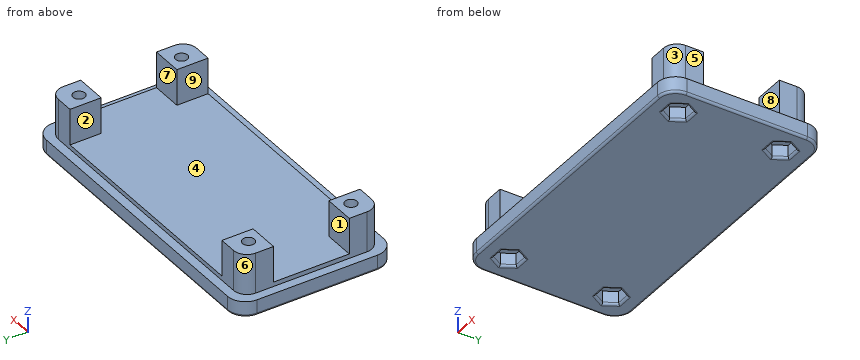
```python
from build123d import *

# Parameters (mm, degrees)
F1_DEPTH = 3.5
F3_DEPTH = 1
F5_DEPTH = 8.1
F6_R     = 1.35
F7_DEPTH = 3
F8_DEPTH = 12.601
F9_R     = 0.5


with BuildPart() as f1:
    # F0 (on Top) → F1 (new body)
    with BuildSketch(Plane.XY):
        with BuildLine():
            Line((31, 17.5), (-31, 17.5))
            ThreePointArc((-31, 17.5), (-33.8284271247, 16.3284271247), (-35, 13.5))
            Line((-35, 13.5), (-35, -13.5))
            ThreePointArc((-35, -13.5), (-33.8284271247, -16.3284271247), (-31, -17.5))
            Line((-31, -17.5), (31, -17.5))
            ThreePointArc((31, -17.5), (33.8284271247, -16.3284271247), (35, -13.5))
            Line((35, -13.5), (35, 13.5))
            ThreePointArc((35, 13.5), (33.8284271247, 16.3284271247), (31, 17.5))
        make_face()
    extrude(amount=F1_DEPTH)

    # F2 (on face) → F3 (join)
    with BuildSketch(Plane.XY.offset(3.5)):
        with BuildLine():
            Line((29.9999990687, 15.5), (-30.0000009313, 15.5))
            ThreePointArc((-30.0000009313, 15.5), (-32.1213212749, 14.6213203436), (-33.0000009313, 12.5))
            Line((-33.0000009313, 12.5), (-33.0000009313, -12.5))
            ThreePointArc((-33.0000009313, -12.5), (-32.1213212749, -14.6213203436), (-30.0000009313, -15.5))
            Line((-30.0000009313, -15.5), (29.9999990687, -15.5))
            ThreePointArc((29.9999990687, -15.5), (32.1213194122, -14.6213203436), (32.9999990687, -12.5))
            Line((32.9999990687, -12.5), (32.9999990687, 12.5))
            ThreePointArc((32.9999990687, 12.5), (32.1213194122, 14.6213203436), (29.9999990687, 15.5))
        make_face()
    extrude(amount=F3_DEPTH)

    # F4 (on face) → F5 (join)
    with BuildSketch(Plane.XY.offset(4.5)):
        with BuildLine():
            Line((-26, 15.5), (-30.0000009313, 15.5))
            ThreePointArc((-30.0000009313, 15.5), (-32.1213212749, 14.6213203436), (-33.0000009313, 12.5))
            Line((-33.0000009313, 12.5), (-33.0000009313, 8.5))
            Line((-33.0000009313, 8.5), (-26, 8.5))
            Line((-26, 8.5), (-26, 15.5))
        make_face()
        with BuildLine():
            Line((-26, -8.5), (-33.0000009313, -8.5))
            Line((-33.0000009313, -8.5), (-33.0000009313, -12.5))
            ThreePointArc((-33.0000009313, -12.5), (-32.1213212749, -14.6213203436), (-30.0000009313, -15.5))
            Line((-30.0000009313, -15.5), (-26, -15.5))
            Line((-26, -15.5), (-26, -8.5))
        make_face()
        with BuildLine():
            Line((29.9999990687, 15.5), (26, 15.5))
            Line((26, 15.5), (26, 8.5))
            Line((26, 8.5), (32.9999990687, 8.5))
            Line((32.9999990687, 8.5), (32.9999990687, 12.5))
            ThreePointArc((32.9999990687, 12.5), (32.1213194122, 14.6213203436), (29.9999990687, 15.5))
        make_face()
        with BuildLine():
            Line((32.9999990687, -12.5), (32.9999990687, -8.5))
            Line((32.9999990687, -8.5), (26, -8.5))
            Line((26, -8.5), (26, -15.5))
            Line((26, -15.5), (29.9999990687, -15.5))
            ThreePointArc((29.9999990687, -15.5), (32.1213194122, -14.6213203436), (32.9999990687, -12.5))
        make_face()
    extrude(amount=F5_DEPTH)

    # F6 (on face) → F7 (cut)
    with BuildSketch(Plane(origin=(0, 0, 0), x_dir=(1, 0, 0), z_dir=(0, 0, -1))):
        Polygon((-30.5011106999, 8.9), (-27.4988893001, 8.9), (-25.9977786002, 11.5), (-27.4988893001, 14.1), (-30.5011106999, 14.1), (-32.0022213998, 11.5), align=None)
        with Locations((-29, 11.5)):
            Circle(F6_R, mode=Mode.SUBTRACT)
        Polygon((27.4988893001, 8.9), (30.5011106999, 8.9), (32.0022213998, 11.5), (30.5011106999, 14.1), (27.4988893001, 14.1), (25.9977786002, 11.5), align=None)
        with Locations((29, 11.5)):
            Circle(F6_R, mode=Mode.SUBTRACT)
        Polygon((30.5011106999, -8.9), (27.4988893001, -8.9), (25.9977786002, -11.5), (27.4988893001, -14.1), (30.5011106999, -14.1), (32.0022213998, -11.5), align=None)
        with Locations((29, -11.5)):
            Circle(F6_R, mode=Mode.SUBTRACT)
        Polygon((-27.4988893001, -8.9), (-30.5011106999, -8.9), (-32.0022213998, -11.5), (-30.5011106999, -14.1), (-27.4988893001, -14.1), (-25.9977786002, -11.5), align=None)
        with Locations((-29, -11.5)):
            Circle(F6_R, mode=Mode.SUBTRACT)
    extrude(amount=-F7_DEPTH, mode=Mode.SUBTRACT)

    # F8 (cut, through all): faces of the model
    f8_faces = [f1.faces().sort_by_distance(p)[0] for p in [
        (-29, -11.5, 0),
        (29, -11.5, 0),
        (29, 11.5, 0),
        (-29, 11.5, 0),
    ]]
    extrude(f8_faces, amount=-F8_DEPTH, mode=Mode.SUBTRACT)

    # F9
    f9_edges = [f1.edges().sort_by_distance(p)[0] for p in [
        (0, 17.5, 0),
        (33.828427, 16.328427, 0),
        (-33.828427, 16.328427, 0),
        (35, 0, 0),
        (-35, 0, 0),
        (33.828427, -16.328427, 0),
        (-33.828427, -16.328427, 0),
        (0, -17.5, 0),
        (-31.251666, -12.8, 0),
        (-29, -14.1, 0),
        (-26.748334, -12.8, 0),
        (-26.748334, -10.2, 0),
        (-29, -8.9, 0),
        (-31.251666, -10.2, 0),
        (26.748334, -10.2, 0),
        (26.748334, -12.8, 0),
        (29, -14.1, 0),
        (31.251666, -12.8, 0),
        (31.251666, -10.2, 0),
        (29, -8.9, 0),
        (-26.748334, 10.2, 0),
        (-26.748334, 12.8, 0),
        (-29, 14.1, 0),
        (-31.251666, 12.8, 0),
        (-31.251666, 10.2, 0),
        (-29, 8.9, 0),
        (31.251666, 10.2, 0),
        (31.251666, 12.8, 0),
        (29, 14.1, 0),
        (26.748334, 12.8, 0),
        (26.748334, 10.2, 0),
        (29, 8.9, 0),
    ]]
    fillet(f9_edges, radius=F9_R)


solid = f1.part
```
Check sheet for the modelled part. Datum: model origin and axes. Units: mm. Face numbers are marked on the shaded views. A direction names the side the tool comes from. Round coordinates to 2 decimals unless told otherwise and drop trailing zeros. Order: outer loops, then holes, each group sorted by start corner. A loop starts at its lowest first (then second) coordinate and runs counter-clockwise, first axis right, second up.
1) Section check C-C (y = 7.5). Record the boundary of the cut face in (x, z).
2) Section check A-A (z = 5.5). Record the boundary of the cut face in (x, y).
3) Mould release check, pull along Y, two halves, no side actions. Record for the marked faces 6, 7, 8 and 9: +Y half, -Y half, draft (parallel to the pull), parting line (faces both ways), or undercut.
4) Scan lines: line 1 (Y direction, x = -29.5, z = 0.5); line 2 (Y direction, x = -29, z = 5.5); line 3 (X direction, y = -11.5, z = 5.75). Record each from-to range of solid material in increasing order.
5) Tool access check on the marked faces 1, 2, 3, 4 and 5. Record the directions out of +Z, -Z, +X, -X, +Y, -Y that give a thin tool (end or side, any length) a straight path to the whole face; none if there is none.
6) Section check B-B (x = -29). Give the number of separate pieces and of enclosed holes in the cut face, and give its area (3 significant figures).
7) Go/stop test with flat-tipped pins: pin 1 Ø2 at (x, z) = (28, 8) entering from -Y; pin 2 Ø2 at (y, z) = (12, 9) entering from +X; pin 3 Ø2.5 at (x, y) = (-27.5, -11.5) entering from -Z. Record where each tip stops, or that it passes through.
Result:
1. outline: (-35, 0.5) arc R0.5 ccw to (-34.5, 0) - (34.5, 0) arc R0.5 ccw to (35, 0.5) - (35, 3.5) - (33, 3.5) - (33, 4.5) - (-33, 4.5) - (-33, 3.5) - (-35, 3.5) - close
2. outline: (-33, -12.5) arc R3 ccw to (-30, -15.5) - (-26, -15.5) - (-26, -8.5) - (-33, -8.5) - close; (-33, 8.5) - (-26, 8.5) - (-26, 15.5) - (-30, 15.5) arc R3 ccw to (-33, 12.5) - close; (26, -15.5) - (30, -15.5) arc R3 ccw to (33, -12.5) - (33, -8.5) - (26, -8.5) - close; (26, 8.5) - (33, 8.5) - (33, 12.5) arc R3 ccw to (30, 15.5) - (26, 15.5) - close; hole circle Ø2.7 at (-29, -11.5); hole circle Ø2.7 at (-29, 11.5); hole circle Ø2.7 at (29, -11.5); hole circle Ø2.7 at (29, 11.5)
3. face 6: +Y half
3. face 7: undercut
3. face 8: undercut
3. face 9: draft
4. line 1: y = -17.5 to -14.1, -8.9 to 8.9, 14.1 to 17.5
4. line 2: y = -15.5 to -12.85, -10.15 to -8.5, 8.5 to 10.15, 12.85 to 15.5
4. line 3: x = -33 to -30.35, -27.65 to -26, 26 to 27.65, 30.35 to 33
5. face 1: +Z, +X, -X
5. face 2: +Z, +Y, -Y
5. face 3: +Z, +X, -Y
5. face 4: +Z
5. face 5: +Z, +X, +Y, -Y
6. separate pieces: 3
6. enclosed holes: 0
6. area: 184 mm2
7. pin 1: stops at y = -15.5
7. pin 2: stops at x = 33
7. pin 3: stops at z = 3
